Can you work these out from the model? Positions are in its coordinate system, mm. Round coordinates to 2 decimals unless told otherwise and drop trailing zeros. Loops run counter-clockwise (first coordinate to the right, second up) from the corner with the lowest first, then second, coordinate; pieces in that order, holes last. Notation, with made-up numbers: (-30.75, 14.25) -> (-1.75, 14.25) arc R18 ccw to (-1.75, 25.25) -> close; hole circle Ø1 at (4.5, 38.25). An arc over 180 degrees is marked (long way). Write each question's results on one line, items separated by ' | '.
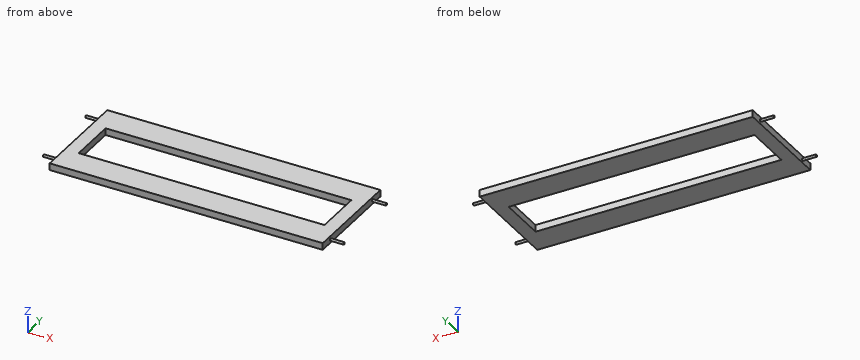
from build123d import *

# Parameters (mm, degrees)
SKETCH013_W             = 400
SKETCH013_H             = 150
SKETCH013_W_2           = 360
SKETCH013_H_2           = 70
PAD013_DEPTH            = 10
CYLINDER013_R           = 1.7
CYLINDER013_DEPTH       = 20
CYLINDER013_PITCH_ANGLE = 90
CYLINDER015_R           = 1.7
CYLINDER015_DEPTH       = 20
CYLINDER015_PITCH_ANGLE = 90
CYLINDER016_R           = 1.7
CYLINDER016_DEPTH       = 20
CYLINDER016_PITCH_ANGLE = 90
CYLINDER017_R           = 1.7
CYLINDER017_DEPTH       = 20
CYLINDER017_PITCH_ANGLE = 90


with BuildPart() as pad013:
    # Sketch013 → Pad013 (new body)
    with BuildSketch(Plane(origin=(0, -10, 60), x_dir=(1, 0, 0), z_dir=(0, 0, 1))):
        Rectangle(SKETCH013_W, SKETCH013_H)
        Rectangle(SKETCH013_W_2, SKETCH013_H_2, mode=Mode.SUBTRACT)
    extrude(amount=PAD013_DEPTH)


with BuildPart() as cylinder013:
    # Cylinder013 → Cylinder013 (new body)
    with BuildSketch(Plane.XY):
        Circle(CYLINDER013_R)
    extrude(amount=CYLINDER013_DEPTH)


with BuildPart() as cylinder013_1:
    # Cylinder013 pitch: moved
    add(cylinder013.part.rotate(Axis((0, 0, 0), (0, 1, 0)), CYLINDER013_PITCH_ANGLE))


with BuildPart() as cylinder013_2:
    # Cylinder013 placement: moved
    add(cylinder013_1.part.moved(Location((200, -65, 65))))


with BuildPart() as cylinder015:
    # Cylinder015 → Cylinder015 (new body)
    with BuildSketch(Plane.XY):
        Circle(CYLINDER015_R)
    extrude(amount=CYLINDER015_DEPTH)


with BuildPart() as cylinder015_1:
    # Cylinder015 pitch: moved
    add(cylinder015.part.rotate(Axis((0, 0, 0), (0, 1, 0)), CYLINDER015_PITCH_ANGLE))


with BuildPart() as cylinder015_2:
    # Cylinder015 placement: moved
    add(cylinder015_1.part.moved(Location((-220, -65, 65))))


with BuildPart() as cylinder016:
    # Cylinder016 → Cylinder016 (new body)
    with BuildSketch(Plane.XY):
        Circle(CYLINDER016_R)
    extrude(amount=CYLINDER016_DEPTH)


with BuildPart() as cylinder016_1:
    # Cylinder016 pitch: moved
    add(cylinder016.part.rotate(Axis((0, 0, 0), (0, 1, 0)), CYLINDER016_PITCH_ANGLE))


with BuildPart() as cylinder016_2:
    # Cylinder016 placement: moved
    add(cylinder016_1.part.moved(Location((-220, 45, 65))))


with BuildPart() as fusion005:
    # Cylinder017 → Cylinder017 (new body)
    with BuildSketch(Plane.XY):
        Circle(CYLINDER017_R)
    extrude(amount=CYLINDER017_DEPTH)


with BuildPart() as fusion005_1:
    # Cylinder017 pitch: moved
    add(fusion005.part.rotate(Axis((0, 0, 0), (0, 1, 0)), CYLINDER017_PITCH_ANGLE))


with BuildPart() as fusion005_2:
    # Cylinder017 placement: moved
    add(fusion005_1.part.moved(Location((200, 45, 65))))

    # Fusion004: union Cylinder013, Cylinder015, Cylinder016
    add(cylinder013_2.part)
    add(cylinder015_2.part)
    add(cylinder016_2.part)

    # Fusion005: union Pad013
    add(pad013.part)


solid = fusion005_2.part
1. If we section it at B-B (y = -1): List the corners of the cut face in (x, z) for me.
Final values:
outline: (-200, 60) -> (-180, 60) -> (-180, 70) -> (-200, 70) -> close; (180, 60) -> (200, 60) -> (200, 70) -> (180, 70) -> close
2. If we section it at D-D (y = -49.5): List the corners of the cut face in (x, z) for me, then the cut area to 3 significant figures.
Final values:
outline: (-200, 60) -> (200, 60) -> (200, 70) -> (-200, 70) -> close | area: 4,000 mm2
3. Will these pins go through, and if not, where does the flat tip stop? pin 1 (3 mm diameter, centred on y = -8, z = 64, fed in from -X); pin 2 (3 mm diameter, centred on y = -12, z = 67.5, fed in from +X).
Final values:
pin 1: x = -200 | pin 2: x = 200
4. If we section it at C-C (z = 65): List the corners of the cut face in (x, y) for me, then the cut area to 3 significant figures.
Final values:
outline: (-220, -66.7) -> (-200, -66.7) -> (-200, -85) -> (200, -85) -> (200, -66.7) -> (220, -66.7) -> (220, -63.3) -> (200, -63.3) -> (200, 43.3) -> (220, 43.3) -> (220, 46.7) -> (200, 46.7) -> (200, 65) -> (-200, 65) -> (-200, 46.7) -> (-220, 46.7) -> (-220, 43.3) -> (-200, 43.3) -> (-200, -63.3) -> (-220, -63.3) -> close; hole (-180, -45) -> (180, -45) -> (180, 25) -> (-180, 25) -> close | area: 35,100 mm2
5. Please list where these lines run through material, in increasing order: line 1 (Y direction, x = -157, z = 63.75); line 2 (X direction, y = -4.5, z = 68.25); line 3 (X direction, y = 49.5, z = 65.5). Write a range as from..to.
Final values:
line 1: -85..-45, 25..65 | line 2: -200..-180, 180..200 | line 3: -200..200
6. If we section it at A-A (x = 92): List the corners of the cut face in (y, z) for me.
Final values:
outline: (-85, 60) -> (-45, 60) -> (-45, 70) -> (-85, 70) -> close; (25, 60) -> (65, 60) -> (65, 70) -> (25, 70) -> close
